Design review of the part built by this model. Coordinates are the model's own, in mm. Face numbers are marked on the shaded views. A direction names the side the tool comes from. Coordinates: 2 decimals unless noted, no trailing zeros. Write each loop counter-clockwise with the first axis right and the second up, starting at its lowest first coordinate (ties: lowest second). Pieces come first, ordered by that corner, then holes. Notation, with made-up numbers: (-37, 37) -> (-7, 37) arc R19 ccw to (-7, 52) -> close; hole circle Ø6 at (53, 20). An arc over 180 degrees is marked (long way). Write item = value, one per line. Start each with the question number.
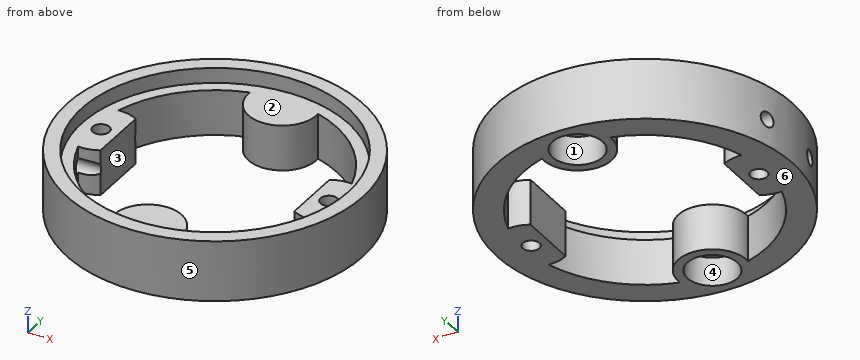
```python
from build123d import *

# Parameters (mm, degrees)
F0_R      = 19.5
F1_DEPTH  = 8
F2_R      = 17.55
F3_DEPTH  = 2
F5_DEPTH  = 6
F6_R      = 1.1
F7_DEPTH  = 6
F8_R      = 3.3
F9_DEPTH  = 3.75
F10_R     = 1
F11_DEPTH = 25
F12_W     = 3.246098
F12_H     = 10.70335
F13_DEPTH = 6


with BuildPart() as f1:
    # F0 (on Top) → F1 (new body)
    with BuildSketch(Plane.XY):
        Circle(F0_R)
    extrude(amount=F1_DEPTH)

    # F2 (on face) → F3 (cut)
    with BuildSketch(Plane.XY.offset(8)):
        Circle(F2_R)
    extrude(amount=-F3_DEPTH, mode=Mode.SUBTRACT)

    # F4 (on face) → F5 (cut)
    with BuildSketch(Plane.XY.offset(6)):
        with BuildLine():
            ThreePointArc((15.358333, -4.48571), (10.5, 0), (15.358333, 4.48571))
            ThreePointArc((15.358333, 4.48571), (11.313708, 11.313708), (4.48571, 15.358333))
            ThreePointArc((4.48571, 15.358333), (0, 10.5), (-4.48571, 15.358333))
            ThreePointArc((-4.48571, 15.358333), (-11.313708, 11.313708), (-15.358333, 4.48571))
            ThreePointArc((-15.358333, 4.48571), (-10.5, 0), (-15.358333, -4.48571))
            ThreePointArc((-15.358333, -4.48571), (-11.313708, -11.313708), (-4.48571, -15.358333))
            ThreePointArc((-4.48571, -15.358333), (0, -10.5), (4.48571, -15.358333))
            ThreePointArc((4.48571, -15.358333), (11.313708, -11.313708), (15.358333, -4.48571))
        make_face()
    extrude(amount=-F5_DEPTH, mode=Mode.SUBTRACT)

    # F6 (on face) → F7 (cut)
    with BuildSketch(Plane.XY.offset(6)):
        with Locations((-15, 0)):
            Circle(F6_R)
        with Locations((15, 0)):
            Circle(F6_R)
    extrude(amount=-F7_DEPTH, mode=Mode.SUBTRACT)

    # F8 (on Top) → F9 (cut)
    with BuildSketch(Plane.XY):
        with Locations((0, 15)):
            Circle(F8_R)
        with Locations((0, -15)):
            Circle(F8_R)
    extrude(amount=F9_DEPTH, mode=Mode.SUBTRACT)

    # F10 (on Right) → F11 (cut)
    with BuildSketch(Plane.YZ):
        with Locations((-4.74, 3.502372)):
            Circle(F10_R)
        with Locations((4.74, 3.502372)):
            Circle(F10_R)
    extrude(amount=-F11_DEPTH, mode=Mode.SUBTRACT)

    # F12 (on face) → F13 (cut)
    with BuildSketch(Plane.XY.offset(6)):
        with Locations((-11.142012, -0.109914)):
            Rectangle(F12_W, F12_H)
        with Locations((11.142012, -0.109914)):
            Rectangle(F12_W, F12_H)
    extrude(amount=-F13_DEPTH, mode=Mode.SUBTRACT)


solid = f1.part
```
(1) Take a section at C-C, the plane y = -13.5. State the section outline as (x, z) points, then the cut area to 3 significant figures.
(2) Take a section at D-D, the plane x = 7.5. State the section outline as (y, z) points.
(3) For line 1 (Y direction, x = 0, z = 2.35); line 2 (X direction, y = -14, z = 2); line 3 (Y direction, x = -17, z = 3), list the stretches that pass through material, from the lowest coordinate up.
(4) Mouldability with a two-part tool opening along X and no side actions: class the marked faces 4, 5 and 6 as pulls with the +X half, pulls with the -X half, needs draft (parallel to the pull), parting line crosses it, or undercut.
(5) Take a section at A-A, the plane x = 0. State the section outline as (y, z) points, then the cut area to 3 significant figures.
(6) Take a section at B-B, the plane z = 5.5. State the section outline as (x, y) points.
(7) For the marked faces 1, 2 and 3, list the 3-axis set-ups (+Z, -Z, +X, -X, +Y, -Y) from which the entire face can be reached by the end or side of a thin tool; tool diameter is ignored.
(8) For pin 1 Ø2 at (x, z) = (15, 5) entering from -Y; pin 2 Ø3 at (x, y) = (-15, 0) entering from +Z; pin 3 Ø1.8 at (y, z) = (-4.74, 3.5) entering from +X, all flat-tipped, find the tip position at first contact; note any pin that passes through.
Report:
q1.outline = (-14.07, 0) -> (-8.59, 0) -> (-8.59, 6) -> (-11.21, 6) -> (-11.21, 8) -> (-14.07, 8) -> close; (-4.24, 0) -> (-2.94, 0) -> (-2.94, 3.75) -> (2.94, 3.75) -> (2.94, 0) -> (4.24, 0) -> (4.24, 6) -> (-4.24, 6) -> close; (8.59, 0) -> (14.07, 0) -> (14.07, 8) -> (11.21, 8) -> (11.21, 6) -> (8.59, 6) -> close
q1.area = 106 mm2
q2.outline = (-18, 0) -> (-14.13, 0) -> (-14.13, 6) -> (-15.87, 6) -> (-15.87, 8) -> (-18, 8) -> close; (14.13, 0) -> (18, 0) -> (18, 8) -> (15.87, 8) -> (15.87, 6) -> (14.13, 6) -> close
q3.line_1 = -19.5 to -18.3, -11.7 to -10.5, 10.5 to 11.7, 18.3 to 19.5
q3.line_2 = -13.57 to -7.75, -4.39 to -3.14, 3.14 to 4.39, 7.75 to 13.57
q3.line_3 = -9.55 to -5.6, -3.88 to 3.88, 5.6 to 9.55
q4.face_4 = undercut
q4.face_5 = parting line crosses it
q4.face_6 = needs draft
q5.outline = (-19.5, 0) -> (-18.3, 0) -> (-18.3, 3.75) -> (-11.7, 3.75) -> (-11.7, 0) -> (-10.5, 0) -> (-10.5, 6) -> (-17.55, 6) -> (-17.55, 8) -> (-19.5, 8) -> close; (10.5, 0) -> (11.7, 0) -> (11.7, 3.75) -> (18.3, 3.75) -> (18.3, 0) -> (19.5, 0) -> (19.5, 8) -> (17.55, 8) -> (17.55, 6) -> (10.5, 6) -> close
q5.area = 66.3 mm2
q6.outline = circle Ø39 at (0, 0); hole circle Ø2.2 at (-15, 0); hole (-15.36, -4.49) arc R16 ccw to (-4.49, -15.36) arc R4.5 cw (long way) to (4.49, -15.36) arc R16 ccw to (15.36, -4.49) arc R4.5 cw to (12.77, -3.91) -> (12.77, 3.91) arc R4.5 cw to (15.36, 4.49) arc R16 ccw to (4.49, 15.36) arc R4.5 cw (long way) to (-4.49, 15.36) arc R16 ccw to (-15.36, 4.49) arc R4.5 cw to (-12.77, 3.91) -> (-12.77, -3.91) arc R4.5 cw to start; hole circle Ø2.2 at (15, 0)
q7.face_1 = -Z
q7.face_2 = +Z
q7.face_3 = +Z, -Z
q8.pin_1 = -13.57
q8.pin_2 = 6
q8.pin_3 = 19.12
